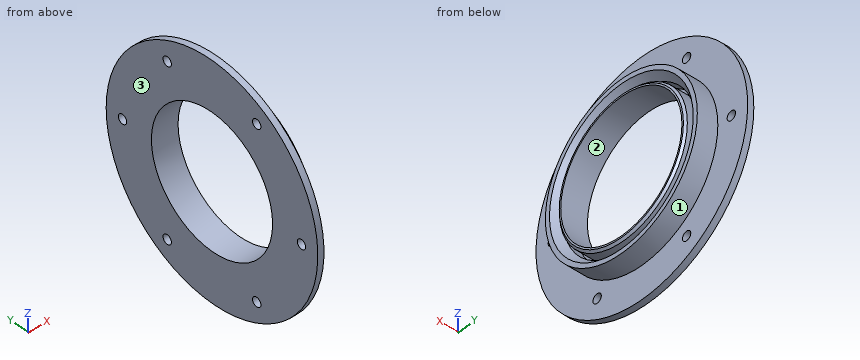
from build123d import *

# Parameters (mm, degrees)
CHAMFER1_SIZE      = 4
CHAMFER1_SIZE2     = 2.800830153
CHAMFER2_SIZE      = 1
SKETCH2_R          = 2.25
CUT_EXTRUDE1_DEPTH = 10
CIRPATTERN1_COUNT  = 6


with BuildPart() as part:
    # Sketch1 → Revolve1 (revolve)
    with BuildSketch(Plane.XY):
        Polygon((0, 32.5), (13, 32.5), (13, 34.3), (3, 34.3), (3, 35.75), (13, 35.75), (13, 40.75), (3, 40.75), (3, 56.75), (0, 56.75), align=None)
    revolve(axis=Axis((0, 0, 0), (1, 0, 0)))

    # Chamfer1
    chamfer1_edges = [part.edges().sort_by_distance(p)[0] for p in [
        (13, -35.75, 0),
    ]]
    chamfer1_side = [part.faces().sort_by_distance(p)[0] for p in [
        (8, -35.75, 0),
    ]]
    chamfer(chamfer1_edges, length=CHAMFER1_SIZE, length2=CHAMFER1_SIZE2, reference=chamfer1_side[0])

    # Chamfer2
    chamfer2_edges = [part.edges().sort_by_distance(p)[0] for p in [
        (13, -34.3, 0),
    ]]
    chamfer(chamfer2_edges, length=CHAMFER2_SIZE)

    # Sketch2 → Cut-Extrude1 (cut)
    with BuildSketch(Plane(origin=(3, 0, 0), x_dir=(0, 0, -1), z_dir=(1, 0, 0))):
        with Locations((0, 48)):
            Circle(SKETCH2_R)
    cut_extrude1 = extrude(amount=-CUT_EXTRUDE1_DEPTH, mode=Mode.SUBTRACT)

    # CirPattern1: Cut-Extrude1 ×6 about axis
    cirpattern1_axis = Axis((0, 0, 0), (1, 0, 0))
    for i in range(1, CIRPATTERN1_COUNT):
        add(cut_extrude1.rotate(cirpattern1_axis, i * 360 / CIRPATTERN1_COUNT), mode=Mode.SUBTRACT)


solid = part.part
Model file for the job. Use its own axes, mm. Face numbers are marked on the shaded views. Give positions to 0.01 mm unless a question says otherwise; leave off trailing zeros. Order: outer loops, then holes, each group sorted by start corner. A loop starts at its lowest first (then second) coordinate and runs counter-clockwise, first axis right, second up. Notation, with made-up numbers: (18, 62.5) - (25, 62.5) arc R20 cw to (25, 80.5) - close; hole circle Ø9 at (49, 85.25). An arc over 180 degrees is marked (long way). Return JSON: item names as keys, results as strings.
1) Pull direction Z, two halves, no side cores. Call the marked faces 1, 2 and 3: pulls with the +Z half, pulls with the -Z half, needs draft (parallel to the pull), parting line crosses it, or undercut.
Geometry says:
{"face 1": "parting line crosses it", "face 2": "undercut", "face 3": "needs draft"}
2) Probe line 1 (Z direction, x = 7.25, y = 0); line 2 (Z direction, x = 10, y = 0); line 3 (Y direction, x = 5.25, z = -11). List the from-to ranges inside material, lowest first. Write a range as from..to.
Geometry says:
{"line 1": "-40.75..-35.75, -34.3..-32.5, 32.5..34.3, 35.75..40.75", "line 2": "-40.75..-36.45, -34.3..-32.5, 32.5..34.3, 36.45..40.75", "line 3": "-39.24..-34.02, -32.49..-30.58, 30.58..32.49, 34.02..39.24"}
3) Cut at B-B, the plane y = 0. Give the cut face in (x, z), plus the area to 3 significant figures.
Geometry says:
{"outline": "(0, -56.75) - (3, -56.75) - (3, -40.75) - (13, -40.75) - (13, -38.55) - (9, -35.75) - (3, -35.75) - (3, -34.3) - (12, -34.3) - (13, -33.3) - (13, -32.5) - (0, -32.5) - close; (0, 32.5) - (13, 32.5) - (13, 33.3) - (12, 34.3) - (3, 34.3) - (3, 35.75) - (9, 35.75) - (13, 38.55) - (13, 40.75) - (3, 40.75) - (3, 56.75) - (0, 56.75) - close", "area": "269 mm²"}
4) Cut at C-C, the plane x = 5.25. Give the cut face in (y, z), plus the area to 3 significant figures.
Geometry says:
{"outline": "circle Ø81.5 at (0, 0); circle Ø68.6 at (0, 0); hole circle Ø71.5 at (0, 0); hole circle Ø65 at (0, 0)", "area": "1,580 mm²"}
5) Flat gauge pins, fed straight in: P1, Ø1, axis at x = 9, y = 31.5, coming from the +Z side; P2, Ø4, axis at x = 3.5, y = -9.5, coming from the -Z side; P3, Ø2.5, axis at y = 24, z = -41.57, coming from the -X side; P4, Ø7, axis at y = -24, z = 41.57, coming from the +X side. Where does each tip first touch, or does it go through?
Geometry says:
{"P1": "z = 26.45", "P2": "z = -56.24", "P3": "through", "P4": "x = 3"}
6) Cut at A-A, the plane z = 0. Count the separate pieces of the cut face and the enclosed holes in it, plus the area to 3 significant figures.
Geometry says:
{"separate pieces": "4", "enclosed holes": "0", "area": "242 mm²"}
7) Cut at D-D, the plane y = 48. Give the cut face in (x, z), plus the area to 3 significant figures.
Geometry says:
{"outline": "(0, -30.27) - (3, -30.27) - (3, -2.25) - (0, -2.25) - close; (0, 2.25) - (3, 2.25) - (3, 30.27) - (0, 30.27) - close", "area": "168 mm²"}
